Check sheet for the drawn part. Datum: minimum x, y, z corner. Units: mm. A direction names the side the tool comes from. Coordinates: 2 decimals unless noted, no trailing zeros. Loops run counter-clockwise (first coordinate to the right, second up) from the corner with the lowest first, then second, coordinate; pieces in that order, holes last.
Q1. Sectioned sample at C-C (x = 40). Enter the section's corners in (y, z) (1 decimal), then the cut area to 3 significant figures.
Q2. Sectioned sample at B-B (z = 35). Enter the section's corners in (x, y) (1 decimal).
Q3. Sectioned sample at A-A (y = 16). Enter the section's corners in (x, z), then the cut area to 3 significant figures.
Q4. Sectioned sample at D-D (y = 11). Enter the section's corners in (x, z).
Q5. Go/stop test with flat-tipped pins: P1, Ø11, axis at x = 26, y = 8.5, coming from the +Z side; P2, Ø5, axis at x = 20, z = 35, coming from the -Y side. Record where each tip stops, or that it passes through.
Q6. Material ranges on probe 1 along X at (y, z) = (6, 2); probe 2 along Y at (x, z) = (7, 2); probe 3 along X at (y, z) = (11, 1.2), recorded low to high.
Q7. Access from +Z, -Z, +X, -X, +Y, -Y to the whole of each face (thin tool, end or side, straight path). Record for the marked faces 1 and 2.
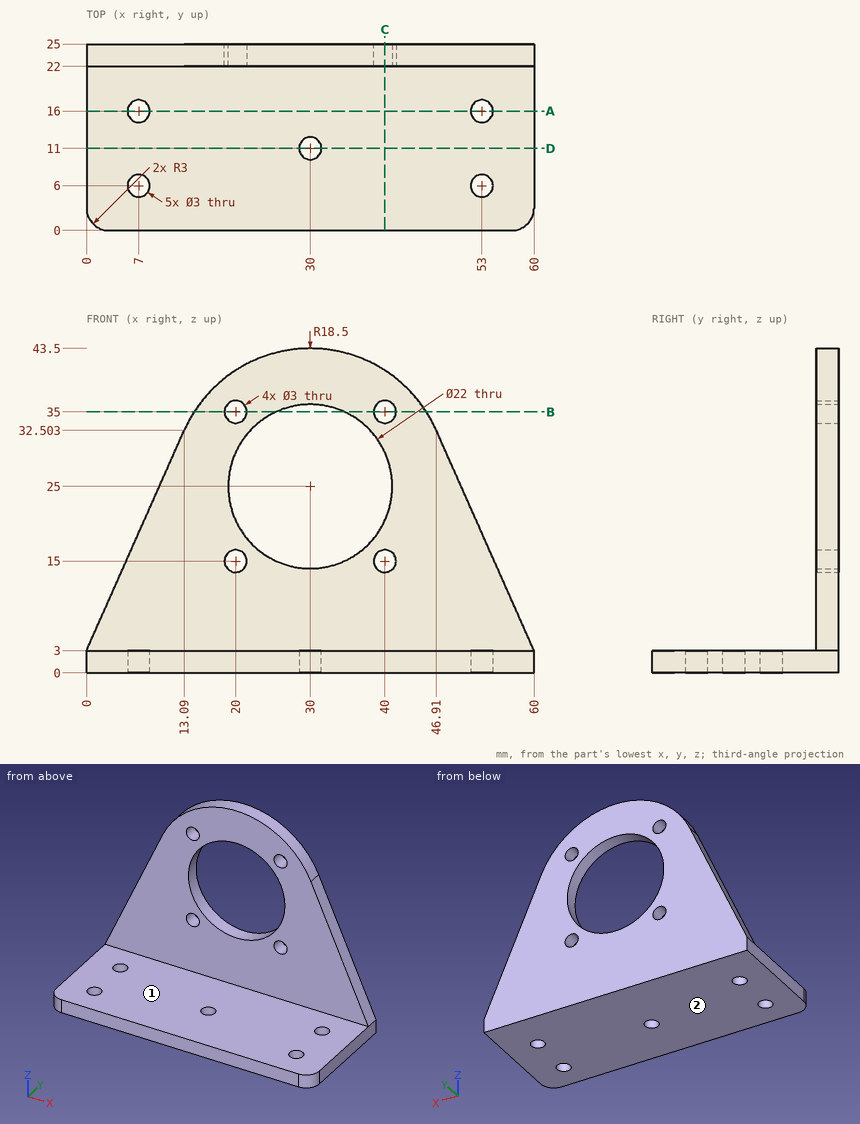
Geometry check:
1. outline: (0, 0) - (25, 0) - (25, 13.5) - (22, 13.5) - (22, 3) - (0, 3) - close; (22, 16.5) - (25, 16.5) - (25, 20.4) - (22, 20.4) - close; (22, 29.6) - (25, 29.6) - (25, 33.5) - (22, 33.5) - close; (22, 36.5) - (25, 36.5) - (25, 40.6) - (22, 40.6) - close
1. area: 142 mm2
2. outline: (14.4, 22) - (18.5, 22) - (18.5, 25) - (14.4, 25) - close; (21.5, 22) - (25.4, 22) - (25.4, 25) - (21.5, 25) - close; (34.6, 22) - (38.5, 22) - (38.5, 25) - (34.6, 25) - close; (41.5, 22) - (45.6, 22) - (45.6, 25) - (41.5, 25) - close
3. outline: (0, 0) - (5.5, 0) - (5.5, 3) - (0, 3) - close; (8.5, 0) - (51.5, 0) - (51.5, 3) - (8.5, 3) - close; (54.5, 0) - (60, 0) - (60, 3) - (54.5, 3) - close
3. area: 162 mm2
4. outline: (0, 0) - (28.5, 0) - (28.5, 3) - (0, 3) - close; (31.5, 0) - (60, 0) - (60, 3) - (31.5, 3) - close
5. P1: stops at z = 3
5. P2: stops at y = 22
6. probe 1: x = 0 to 5.5, 8.5 to 51.5, 54.5 to 60
6. probe 2: y = 0 to 4.5, 7.5 to 14.5, 17.5 to 25
6. probe 3: x = 0 to 28.5, 31.5 to 60
7. face 1: +Z, +X, -X, -Y
7. face 2: -Z, +X, -X, +Y, -Y
